Input: part model. Units: mm. Frame: model coordinates. Face numbers are marked on the shaded views. Coordinates: 2 decimals unless noted, no trailing zeros. Order: outer loops, then holes, each group sorted by start corner. A loop starts at its lowest first (then second) coordinate and runs counter-clockwise, first axis right, second up.
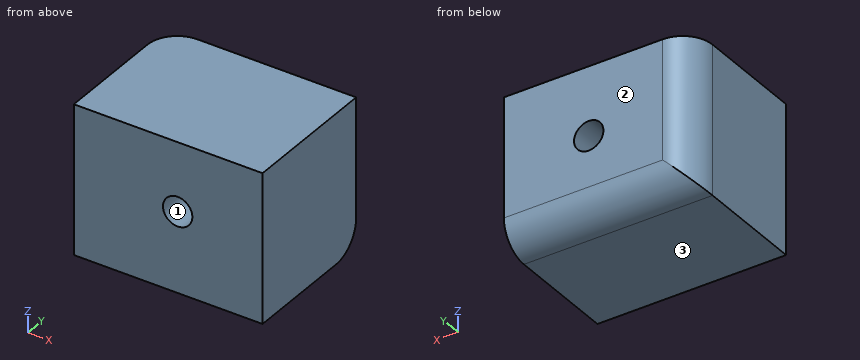
from build123d import *

# Parameters (mm, degrees)
F0_W     = 32.118473202
F0_H     = 23.727130854
F1_DEPTH = 25.4
F2_R     = 5.08
F4_D     = 5


with BuildPart() as f1:
    # F0 (on Top) → F1 (new body)
    with BuildSketch(Plane.XY):
        with Locations((16.059236601, 11.863565427)):
            Rectangle(F0_W, F0_H)
    extrude(amount=F1_DEPTH)

    # F2
    f2_edges = [f1.edges().sort_by_distance(p)[0] for p in [
        (0, 23.727131, 12.7),
        (16.059237, 23.727131, 0),
    ]]
    fillet(f2_edges, radius=F2_R)

    # F4 (through all)
    with Locations(Plane(origin=(0, 23.727130854, 0), x_dir=(-1, 0, 0), z_dir=(0, 1, 0))):
        with Locations((-17.6689904183, 13.7012554333)):
            Hole(F4_D / 2)


solid = f1.part
Item 1: Cut plane A-A on x = 17. Return loops of the section in (y, z), then the cut area to 3 significant figures.
Response values:
outline: (0, 0) - (18.65, 0) arc R5.08 ccw to (23.73, 5.08) - (23.73, 11.29) - (0, 11.29) - close; (0, 16.11) - (23.73, 16.11) - (23.73, 25.4) - (0, 25.4) - close
area: 483 mm2
Item 2: Cut plane B-B on y = 10.75. Return loops of the section in (x, z), then the cut area to 3 significant figures.
Response values:
outline: (0, 0) - (32.12, 0) - (32.12, 25.4) - (0, 25.4) - close; hole circle Ø5 at (17.67, 13.7)
area: 796 mm2
Item 3: Cut plane C-C on z = 2. Return loops of the section in (x, y), then the cut area to 3 significant figures.
Response values:
outline: (0, 0) - (32.12, 0) - (32.12, 22.69) - (2, 22.69) arc R5.08 ccw to (0, 18.65) - close
area: 726 mm2
Item 4: Draft query along Z for the marked faces 1, 2 and 3. Return one class per face: pulls with the +Z half, pulls with the -Z half, needs draft (parallel to the pull), parting line crosses it, or undercut.
Response values:
face 1: undercut
face 2: needs draft
face 3: pulls with the -Z half
Item 5: Ray query, probe 1 along Z at (x, y) = (18, 5.25); probe 2 along Y at (x, z) = (3, 23.75); probe 3 along Z at (x, y) = (21, 20.5). Return the intervals inside material, ascending.
Response values:
probe 1: z = 0 to 11.22, 16.18 to 25.4
probe 2: y = 0 to 23.28
probe 3: z = 0.35 to 25.4
